Autodesk Inventor part; units mm, degrees
ref_plane "YZ Plane" through (0, 0, 0) normal (1, 0, 0) x (0, 1, 0)
ref_plane "XZ Plane" through (0, 0, 0) normal (0, 1, 0) x (-1, 0, 0)
ref_plane "XY Plane" through (0, 0, 0) normal (0, 0, 1) x (1, 0, 0)
sketch "Sketch1" plane through (0, 0, 0) normal (0, 1, 0) x (-1, 0, 0)
  line L0 (-8, -10) -> (8, -10)
  line L1 (10, -8) -> (10, 8)
  line L2 (8, 10) -> (-8, 10)
  line L3 (-10, 8) -> (-10, -8)
  line L4 (-10, -10) -> (10, 10) construction
  line L5 (10, -10) -> (-10, 10) construction
  line L6 (-6, -8) -> (6, -8)
  line L7 (8, -6) -> (8, 6)
  line L8 (6, 8) -> (-6, 8)
  line L9 (-8, 6) -> (-8, -6)
  line L10 (-8, -8) -> (8, 8) construction
  line L11 (8, -8) -> (-8, 8) construction
  arc A0 (10, 8) -> (8, 10) centre (8, 8) ccw
  arc A1 (8, 6) -> (6, 8) centre (6, 6) ccw
  arc A2 (8, -10) -> (10, -8) centre (8, -8) ccw
  arc A3 (6, -8) -> (8, -6) centre (6, -6) ccw
  arc A4 (-10, -8) -> (-8, -10) centre (-8, -8) ccw
  arc A5 (-8, -6) -> (-6, -8) centre (-6, -6) ccw
  arc A6 (-6, 8) -> (-8, 6) centre (-6, 6) ccw
  arc A7 (-8, 10) -> (-10, 8) centre (-8, 8) ccw
  point P0 (0, 0)
  dimension "width" = 20
  dimension "depth" = 20
  dimension "thickness" = 2
  dimension "d3" = 2
extrude "Extrusion1" add sketch "Sketch1" along normal blind 100
equation "\"d3\" = thickness"
properties part number "beam 20x20x2" material "Steel"
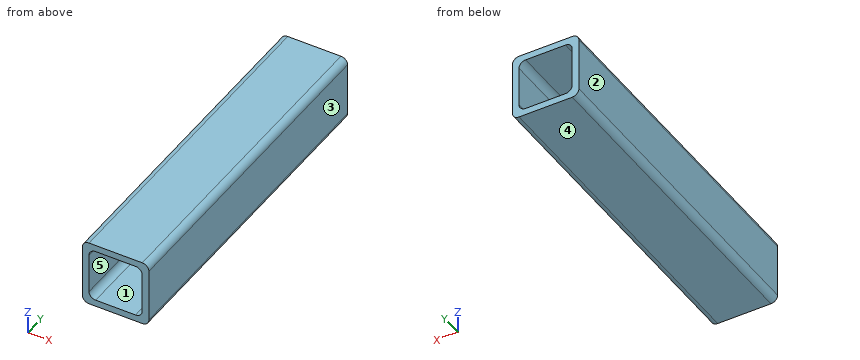
For this review, take the finished solid that the model builds, in its own axes (mm). Face numbers are marked on the shaded views. A direction names the side the tool comes from. Give positions to 0.01 mm unless a question says otherwise; leave off trailing zeros. Order: outer loops, then holes, each group sorted by start corner. A loop starts at its lowest first (then second) coordinate and runs counter-clockwise, first axis right, second up. Notation, with made-up numbers: M 62,75.25 L 67,75.25 A4 cw 67,81.25 Z; hole C 34.25,31.5 d11. An arc over 180 degrees is marked long. Answer in a Markdown table with one row per item. Add a question column.
(1) Wall thickness on probe 1 along Z at (x, y) = (-6, 94); probe 2 along Z at (x, y) = (7.5, 64): over which ranges is each line inside the solid? List them lowest first. Write a range as [from, to].
(2) For pin 1 (3 mm diameter, centred on x = 3, z = -5, fed in from -Y), flat-tipped, find the tip position at first contact; note if it passes through.
(3) Consider section B-B on z = 1.75. State the section outline as (x, y) points.
(4) Mouldability with a two-part tool opening along X and no side actions: class the marked faces 1, 2 and 3 as +X half, -X half, draft (parallel to the pull), parting line (faces both ways), or undercut.
(5) For the marked faces 4 and 5, list the 3-axis set-ups (+Z, -Z, +X, -X, +Y, -Y) from which the entire face can be reached by the end or side of a thin tool; tool diameter is ignored.
(6) Consider section C-C on y = 82. State the section outline as (x, z) points.
(7) Consider section A-A on x = 3.5. State the section outline as (y, z) points, and give its area (3 significant figures).
Evaluation:
| question | item | result |
|---|---|---|
| 1 | probe 1 | z = [-10, -8], [8, 10] |
| 1 | probe 2 | z = [-10, -7.32], [7.32, 10] |
| 2 | pin 1 | passes through |
| 3 | outline | M -10,0 L -8,0 L -8,100 L -10,100 Z; M 8,0 L 10,0 L 10,100 L 8,100 Z |
| 4 | face 1 | undercut |
| 4 | face 2 | -X half |
| 4 | face 3 | +X half |
| 5 | face 4 | -Z, +X, -X, +Y, -Y |
| 5 | face 5 | +Y, -Y |
| 6 | outline | M -10,-8 A2 ccw -8,-10 L 8,-10 A2 ccw 10,-8 L 10,8 A2 ccw 8,10 L -8,10 A2 ccw -10,8 Z; hole M -8,-6 A2 ccw -6,-8 L 6,-8 A2 ccw 8,-6 L 8,6 A2 ccw 6,8 L -6,8 A2 ccw -8,6 Z |
| 7 | outline | M 0,-10 L 100,-10 L 100,-8 L 0,-8 Z; M 0,8 L 100,8 L 100,10 L 0,10 Z |
| 7 | area | 400 mm^2 |
